Input: part model. Units: mm. Frame: model coordinates. Face numbers are marked on the shaded views. A direction names the side the tool comes from. Round coordinates to 2 decimals unless told otherwise and drop trailing zeros. Order: outer loops, then holes, each group sorted by start corner. A loop starts at its lowest first (then second) coordinate and runs counter-clockwise, first axis right, second up.
Item 1: Cut plane D-D on z = -29. Output: boundary loops of the cut face in (x, y), then the cut area to 3 significant figures.
Item 2: First-contact query: pin 1 (4 mm diameter, centred on y = 9, z = -18.5, fed in from -X); pin 2 (1 mm diameter, centred on y = 10.5, z = 6.5, fed in from +X); pin 3 (6 mm diameter, centred on y = 14, z = 9.5, fed in from -X). Flat tips, straight axial feed; report the tip coordinate or a pass-through.
Item 3: Reachability of the marked faces 1 and 2 from +Z, -Z, +X, -X, +Y, -Y: full face, straight path, thin tool, end or side. Return the list, or none.
Item 4: Line query: L1, parallel to X at y = 15.9, z = 0; L2, parallel to X at y = 7.15, z = 0; L3, parallel to Y at x = -31, z = -4. Output: solid intervals per line, ascending.
Item 5: Cut plane C-C on y = 13.75. Output: boundary loops of the cut face in (x, z), then the cut area to 3 significant figures.
```python
from build123d import *

# Parameters (mm, degrees)
SKETCH1_W           = 69.8
SKETCH1_H           = 69.8
BOSS_EXTRUDE1_DEPTH = 4.98
SKETCH2_R           = 30
BOSS_EXTRUDE2_DEPTH = 17
SKETCH3_R           = 25.65
CUT_EXTRUDE1_DEPTH  = 19.98
SKETCH4_R           = 24.15
CUT_EXTRUDE3_DEPTH  = 2
CUT_EXTRUDE4_START  = -6
SKETCH5_R           = 27.15
CUT_EXTRUDE4_DEPTH  = 2
CUT_EXTRUDE5_START  = -14
SKETCH5_2_R         = 27.15
CUT_EXTRUDE5_DEPTH  = 2


with BuildPart() as part:
    # Sketch1 → Boss-Extrude1 (new body)
    with BuildSketch(Plane(origin=(0, 0, 0), x_dir=(1, 0, 0), z_dir=(0, 1, 0))):
        Rectangle(SKETCH1_W, SKETCH1_H)
    extrude(amount=-BOSS_EXTRUDE1_DEPTH)

    # Sketch2 → Boss-Extrude2 (add)
    with BuildSketch(Plane(origin=(0, 0, 0), x_dir=(1, 0, 0), z_dir=(0, 1, 0))):
        with Locations(Location((0, 0, 0), (0, 0, 270))):
            Circle(SKETCH2_R)
    extrude(amount=BOSS_EXTRUDE2_DEPTH)

    # Sketch3 → Cut-Extrude1 (cut)
    with BuildSketch(Plane.XZ.offset(4.98)):
        with Locations(Location((0, 0, 0), (0, 0, 270))):
            Circle(SKETCH3_R)
    extrude(amount=-CUT_EXTRUDE1_DEPTH, mode=Mode.SUBTRACT)

    # Sketch4 → Cut-Extrude3 (cut)
    with BuildSketch(Plane(origin=(0, 17, 0), x_dir=(1, 0, 0), z_dir=(0, 1, 0))):
        with Locations(Location((0, 0, 0), (0, 0, 270))):
            Circle(SKETCH4_R)
    extrude(amount=-CUT_EXTRUDE3_DEPTH, mode=Mode.SUBTRACT)

    # Sketch5 → Cut-Extrude4 (cut)
    with BuildSketch(Plane(origin=(0, 17, 0), x_dir=(1, 0, 0), z_dir=(0, 1, 0)).offset(CUT_EXTRUDE4_START)):
        with Locations(Location((0, 0, 0), (0, 0, 270))):
            Circle(SKETCH5_R)
    extrude(amount=-CUT_EXTRUDE4_DEPTH, mode=Mode.SUBTRACT)

    # Sketch5_2 → Cut-Extrude5 (cut)
    with BuildSketch(Plane(origin=(0, 17, 0), x_dir=(1, 0, 0), z_dir=(0, 1, 0)).offset(CUT_EXTRUDE5_START)):
        with Locations(Location((0, 0, 0), (0, 0, 270))):
            Circle(SKETCH5_2_R)
    extrude(amount=-CUT_EXTRUDE5_DEPTH, mode=Mode.SUBTRACT)


solid = part.part
```
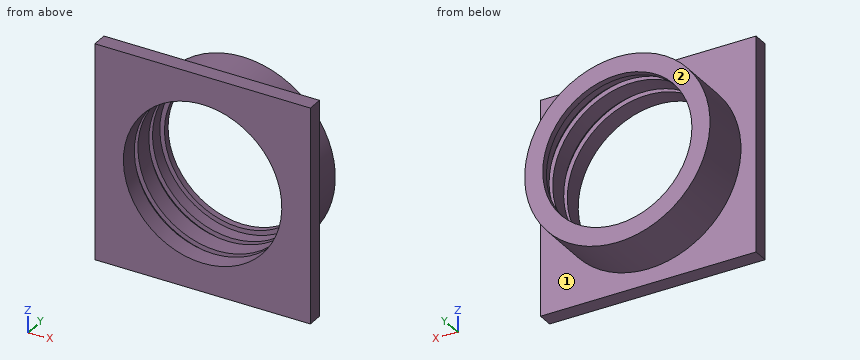
From the geometry:
1. outline: (-34.9, -4.98) - (34.9, -4.98) - (34.9, 0) - (7.68, 0) - (7.68, 17) - (-7.68, 17) - (-7.68, 0) - (-34.9, 0) - close
1. area: 609 mm2
2. pin 1: stops at x = -25.05
2. pin 2: stops at x = 29.39
2. pin 3: stops at x = -29.29
3. face 1: +Y
3. face 2: +Z, -Z, +X, -X, +Y
4. L1: x = -30 to -24.15, 24.15 to 30
4. L2: x = -30 to -25.65, 25.65 to 30
4. L3: y = -4.98 to 0
5. outline: circle Ø60 at (0, 0); hole circle Ø51.3 at (0, 0)
5. area: 761 mm2
